Geometry: final body of the model. Coordinates: model frame, mm. A direction names the side the tool comes from. Round coordinates to 2 decimals unless told otherwise and drop trailing zeros. Answer in a Markdown table with one row per item.
```python
from build123d import *

# Parameters (mm, degrees)
SKETCH_2_R          = 1.5
CUT_EXTRUDE_1_DEPTH = 28
SKETCH_2_4_R        = 3.75
SKETCH_2_4_R_2      = 1.5
CUT_EXTRUDE_2_DEPTH = 1.5
EXTRUDE_START       = 1.5
SKETCH_4_R          = 3.75
SKETCH_4_R_2        = 1.5
EXTRUDE_2_DEPTH     = 1.5
EXTRUDE_START_2     = 0.5
SKETCH_5_R          = 2.359540806
SKETCH_5_R_2        = 1.5
EXTRUDE_3_DEPTH     = 0.5


with BuildPart() as part:
    # 草图1 → 旋转1 (revolve)
    with BuildSketch(Plane(origin=(0, 0, 0), x_dir=(0, 0, -1), z_dir=(1, 0, 0)), mode=Mode.PRIVATE) as revolve_1_sk:
        with BuildLine():
            Line((-14, 4.348576665), (-14, 0))
            Line((-14, 0), (14, 0))
            Line((14, 0), (14, 4.348576665))
            ThreePointArc((14, 4.348576665), (13.741609048, 5.019408999), (13.099967959, 5.343567322))
            ThreePointArc((13.099967959, 5.343567322), (0, 6), (-13.099967959, 5.343567322))
            ThreePointArc((-13.099967959, 5.343567322), (-13.741609048, 5.019408999), (-14, 4.348576665))
        make_face()
    revolve(revolve_1_sk.sketch.rotate(Axis((0, 0, 14), (0, 0, -1)), 90), axis=Axis((0, 0, 14), (0, 0, -1)))

    # 草图2 → 切除-拉伸1 (cut)
    with BuildSketch(Plane.XY.offset(14)):
        Circle(SKETCH_2_R)
    extrude(amount=-CUT_EXTRUDE_1_DEPTH, mode=Mode.SUBTRACT)

    # 草图2<4> → 切除-拉伸2 (cut)
    with BuildSketch(Plane.XY.offset(14)):
        Circle(SKETCH_2_4_R)
        Circle(SKETCH_2_4_R_2, mode=Mode.SUBTRACT)
    cut_extrude_2 = extrude(amount=-CUT_EXTRUDE_2_DEPTH, mode=Mode.SUBTRACT)

    # 镜向1: 切除-拉伸2 across plane
    add(cut_extrude_2.mirror(Plane.XY), mode=Mode.SUBTRACT)

    # 草图4 → 凸台-拉伸2 (add)
    with BuildSketch(Plane.XY.offset(12.5).offset(EXTRUDE_START)):
        Circle(SKETCH_4_R)
        Circle(SKETCH_4_R_2, mode=Mode.SUBTRACT)
    extrude_2 = extrude(amount=-EXTRUDE_2_DEPTH)

    # 草图5 → 凸台-拉伸3 (add)
    with BuildSketch(Plane.XY.offset(14).offset(EXTRUDE_START_2)):
        with Locations(Location((0, 0, 0), (0, 0, 180))):
            Circle(SKETCH_5_R)
        Circle(SKETCH_5_R_2, mode=Mode.SUBTRACT)
    extrude_3 = extrude(amount=-EXTRUDE_3_DEPTH)

    # 镜向4: 凸台-拉伸2, 凸台-拉伸3 across plane
    add(extrude_2.mirror(Plane.XY))
    add(extrude_3.mirror(Plane.XY))


solid = part.part
```
Item 1: Set-up query: faces 1 (the flat face through (2, -2, -14)), 2 (the flat face through (0, 2, 14.5)), 3 (the cylindrical face through (0.31, -2.34, 14.25)). Return all of +Z, -Z, +X, -X, +Y, -Y with unobstructed straight access to the full face (end or side cutting, diameter ignored); none if empty.
Ans:
| item | result |
|---|---|
| face 1 | -Z |
| face 2 | +Z, +X, -X, +Y, -Y |
| face 3 | +Z |
Item 2: Mould query, pull axis Y, two halves, no side actions, for faces 4 (the flat face through (0, 2, -14.5)), 5 (the cylindrical face through (-1.5, 0.07, -0.2)), 6 (the cylindrical face through (0.31, -2.34, -14.25)). Classes: released by +Y, released by -Y, zero draft, split by the parting line, or undercut.
Ans:
| item | result |
|---|---|
| face 4 | zero draft |
| face 5 | undercut |
| face 6 | split by the parting line |
Item 3: First-contact query: P1, Ø6, axis at y = 1.5, z = -10, coming from the +X side; P2, Ø5, axis at x = -4.5, y = -2, coming from the +Z side; P3, Ø1.5, axis at x = -2.5, z = 1.5, coming from the -Y side; P4, Ø5, axis at x = 0, y = 0, coming from the -Z side. Flat tips, straight axial feed; report the tip coordinate or a pass-through.
Ans:
| item | result |
|---|---|
| P1 | x = 5.79 |
| P2 | z = 14 |
| P3 | y = -5.73 |
| P4 | z = -14.5 |
Item 4: Ray query, L1, parallel to Z at x = 1.25, y = 4; L2, parallel to Y at x = 0, z = -6.25; L3, parallel to X at y = -0.5, z = 9. Return the intervals inside material, ascending.
Ans:
| item | result |
|---|---|
| L1 | -14 to 14 |
| L2 | -5.85 to -1.5, 1.5 to 5.85 |
| L3 | -5.67 to -1.41, 1.41 to 5.67 |
